CAD build for the part. Positions are in the model's coordinates, mm. A direction names the side the tool comes from. Coordinates: 2 decimals unless noted, no trailing zeros. Order: outer loops, then holes, each group sorted by start corner. A loop starts at its lowest first (then second) coordinate and runs counter-clockwise, first axis right, second up. Notation, with made-up numbers: (60.25, 24.5) - (95.25, 24.5) arc R9 cw to (95.25, 38.5) - close; hole circle Ø1 at (-37, 33.25). An arc over 180 degrees is marked (long way). Return JSON: item names as keys, results as strings.
from build123d import *

# Parameters (mm, degrees)
F1_R     = 1.5
F2_DEPTH = 3


with BuildPart() as f2:
    # F1 (on Top) → F2 (new body)
    with BuildSketch(Plane.XY):
        Polygon((19.1138070579, -24.5658658908), (30.8861929421, -3.8551877721), (24.5658658908, 19.1138070579), (3.8551877721, 30.8861929421), (-19.1138070579, 24.5658658908), (-30.8861929421, 3.8551877721), (-24.5658658908, -19.1138070579), (-3.8551877721, -30.8861929421), align=None)
        with BuildLine():
            add(Edge.make_bspline(
                [(-4.1445110049, -6.3067241031), (-5.9517399206, -7.2120212694), (-8.2435888807, -7.2120212694)],
                knots=[0, 0, 0, 1, 1, 1], degree=2))
            add(Edge.make_bspline(
                [(-8.2435888807, -7.2120212694), (-10.4546678333, -7.2120212694), (-11.6746314868, -6.0223463687)],
                knots=[0, 0, 0, 1, 1, 1], degree=2))
            add(Edge.make_bspline(
                [(-11.6746314868, -6.0223463687), (-12.8945951403, -4.832671468), (-12.8945951403, -2.665342936)],
                knots=[0, 0, 0, 1, 1, 1], degree=2))
            add(Edge.make_bspline(
                [(-12.8945951403, -2.665342936), (-12.8945951403, -0.49128357), (-12.0263175607, 1.3024836777)],
                knots=[0, 0, 0, 1, 1, 1], degree=2))
            add(Edge.make_bspline(
                [(-12.0263175607, 1.3024836777), (-11.1580399812, 3.0962509255), (-9.6755738036, 4.03688497)],
                knots=[0, 0, 0, 1, 1, 1], degree=2))
            add(Edge.make_bspline(
                [(-9.6755738036, 4.03688497), (-8.193107626, 4.9775190146), (-6.3219357878, 4.9775190146)],
                knots=[0, 0, 0, 1, 1, 1], degree=2))
            add(Edge.make_bspline(
                [(-6.3219357878, 4.9775190146), (-4.4574947836, 4.9775190146), (-3.4175809383, 4.1210203944)],
                knots=[0, 0, 0, 1, 1, 1], degree=2))
            add(Edge.make_bspline(
                [(-3.4175809383, 4.1210203944), (-2.377667093, 3.2645217742), (-2.377667093, 1.7702766373)],
                knots=[0, 0, 0, 1, 1, 1], degree=2))
            add(Edge.make_bspline(
                [(-2.377667093, 1.7702766373), (-2.377667093, -0.1951268762), (-4.1327320455, -1.2619640573)],
                knots=[0, 0, 0, 1, 1, 1], degree=2))
            add(Edge.make_bspline(
                [(-4.1327320455, -1.2619640573), (-5.887796998, -2.3288012385), (-9.148886047, -2.3288012385)],
                knots=[0, 0, 0, 1, 1, 1], degree=2))
            Line((-9.148886047, -2.3288012385), (-9.687352763, -2.3288012385))
            Line((-9.687352763, -2.3288012385), (-9.7075452649, -2.5509187588))
            Line((-9.7075452649, -2.5509187588), (-9.7075452649, -2.7629400283))
            add(Edge.make_bspline(
                [(-9.7075452649, -2.7629400283), (-9.7075452649, -3.7187184492), (-9.1657131319, -4.2706468331)],
                knots=[0, 0, 0, 1, 1, 1], degree=2))
            add(Edge.make_bspline(
                [(-9.1657131319, -4.2706468331), (-8.6238809989, -4.8225752171), (-7.6142559063, -4.8225752171)],
                knots=[0, 0, 0, 1, 1, 1], degree=2))
            add(Edge.make_bspline(
                [(-7.6142559063, -4.8225752171), (-6.6988624891, -4.8225752171), (-5.9517399206, -4.622332907)],
                knots=[0, 0, 0, 1, 1, 1], degree=2))
            add(Edge.make_bspline(
                [(-5.9517399206, -4.622332907), (-5.2046173521, -4.422090597), (-4.1445110049, -3.9172780508)],
                knots=[0, 0, 0, 1, 1, 1], degree=2))
            Line((-4.1445110049, -3.9172780508), (-4.1445110049, -6.3067241031))
        make_face(mode=Mode.SUBTRACT)
        with BuildLine():
            Line((9.8354311099, -0.2994548025), (8.4354176482, -7))
            Line((8.4354176482, -7), (5.2719256916, -7))
            Line((5.2719256916, -7), (6.712324157, -0.1311839537))
            add(Edge.make_bspline(
                [(6.712324157, -0.1311839537), (6.8805950057, 0.582284445), (6.8805950057, 1.1207511611)],
                knots=[0, 0, 0, 1, 1, 1], degree=2))
            add(Edge.make_bspline(
                [(6.8805950057, 1.1207511611), (6.8805950057, 2.4130712795), (5.7430840681, 2.4130712795)],
                knots=[0, 0, 0, 1, 1, 1], degree=2))
            add(Edge.make_bspline(
                [(5.7430840681, 2.4130712795), (4.7772093962, 2.4130712795), (3.9880191156, 1.2133001279)],
                knots=[0, 0, 0, 1, 1, 1], degree=2))
            add(Edge.make_bspline(
                [(3.9880191156, 1.2133001279), (3.1988288349, 0.0135289762), (2.7478629602, -2.1302416369)],
                knots=[0, 0, 0, 1, 1, 1], degree=2))
            Line((2.7478629602, -2.1302416369), (1.7146799488, -7))
            Line((1.7146799488, -7), (-1.4488120078, -7))
            Line((-1.4488120078, -7), (1.0415965538, 4.7587669112))
            Line((1.0415965538, 4.7587669112), (3.461331359, 4.7587669112))
            Line((3.461331359, 4.7587669112), (3.2392138386, 2.5813421283))
            Line((3.2392138386, 2.5813421283), (3.3031567611, 2.5813421283))
            add(Edge.make_bspline(
                [(3.3031567611, 2.5813421283), (4.8377869018, 4.9775190146), (7.0387696036, 4.9775190146)],
                knots=[0, 0, 0, 1, 1, 1], degree=2))
            add(Edge.make_bspline(
                [(7.0387696036, 4.9775190146), (8.4892643198, 4.9775190146), (9.283502726, 4.1008278926)],
                knots=[0, 0, 0, 1, 1, 1], degree=2))
            add(Edge.make_bspline(
                [(9.283502726, 4.1008278926), (10.0777411321, 3.2241367705), (10.0777411321, 1.5919095376)],
                knots=[0, 0, 0, 1, 1, 1], degree=2))
            add(Edge.make_bspline(
                [(10.0777411321, 1.5919095376), (10.0777411321, 0.8245944673), (9.8354311099, -0.2994548025)],
                knots=[0, 0, 0, 1, 1, 1], degree=2))
        make_face(mode=Mode.SUBTRACT)
        with BuildLine():
            add(Edge.make_bspline(
                [(18.7975365148, -5.4754661103), (17.3874268022, -7.2120212694), (15.4422157905, -7.2120212694)],
                knots=[0, 0, 0, 1, 1, 1], degree=2))
            add(Edge.make_bspline(
                [(15.4422157905, -7.2120212694), (13.894123982, -7.2120212694), (13.0056539005, -6.0913374167)],
                knots=[0, 0, 0, 1, 1, 1], degree=2))
            add(Edge.make_bspline(
                [(13.0056539005, -6.0913374167), (12.1171838191, -4.970653564), (12.1171838191, -2.9514033789)],
                knots=[0, 0, 0, 1, 1, 1], degree=2))
            add(Edge.make_bspline(
                [(12.1171838191, -2.9514033789), (12.1171838191, -0.8682102713), (12.8744026385, 1.0197886518)],
                knots=[0, 0, 0, 1, 1, 1], degree=2))
            add(Edge.make_bspline(
                [(12.8744026385, 1.0197886518), (13.6316214579, 2.9077875749), (14.8633640708, 3.9426532947)],
                knots=[0, 0, 0, 1, 1, 1], degree=2))
            add(Edge.make_bspline(
                [(14.8633640708, 3.9426532947), (16.0951066837, 4.9775190146), (17.5657939019, 4.9775190146)],
                knots=[0, 0, 0, 1, 1, 1], degree=2))
            add(Edge.make_bspline(
                [(17.5657939019, 4.9775190146), (18.5855152453, 4.9775190146), (19.3275896884, 4.5366493909)],
                knots=[0, 0, 0, 1, 1, 1], degree=2))
            add(Edge.make_bspline(
                [(19.3275896884, 4.5366493909), (20.0696641314, 4.0957797671), (20.4802450024, 3.2544255233)],
                knots=[0, 0, 0, 1, 1, 1], degree=2))
            Line((20.4802450024, 3.2544255233), (20.5643804267, 3.2544255233))
            Line((20.5643804267, 3.2544255233), (21.1634246483, 4.7587669112))
            Line((21.1634246483, 4.7587669112), (23.6033519553, 4.7587669112))
            Line((23.6033519553, 4.7587669112), (21.0994817258, -7))
            Line((21.0994817258, -7), (18.6898431716, -7))
            Line((18.6898431716, -7), (18.8379215185, -5.4754661103))
            Line((18.8379215185, -5.4754661103), (18.7975365148, -5.4754661103))
        make_face(mode=Mode.SUBTRACT)
        Polygon((-15.8494312445, -7), (-24.4413407821, -7), (-21.1937134011, 8.3765901595), (-17.9730093559, 8.3765901595), (-20.665342936, -4.3076664199), (-15.2806757757, -4.3076664199), align=None, mode=Mode.SUBTRACT)
        with Locations((0, 25)):
            Circle(F1_R, mode=Mode.SUBTRACT)
    extrude(amount=F2_DEPTH)


solid = f2.part
Item 1: Band-saw the part on C-C, the plane y = 14.5. List the corners of the cut face in (x, z), then the cut area to 3 significant figures.
Findings below:
{"outline": "(-24.84, 0) - (25.84, 0) - (25.84, 3) - (-24.84, 3) - close", "area": "152 mm²"}
Item 2: Drop flat-ended pins along their axis: P1, Ø1.2, axis at x = 19.5, z = 1.5, coming from the +Y side; P2, Ø1.5, axis at x = -0.5, z = 2, coming from the +Y side; P3, Ø0.7, axis at x = 22, z = 1, coming from the -Y side. Give the stop position or say it passes through.
Findings below:
{"P1": "stops at y = 22.33", "P2": "stops at y = 29.89", "P3": "stops at y = -20.1"}
Item 3: Band-saw the part on A-A, the plane x = 0. List the corners of the cut face in (y, z), then the cut area to 3 significant figures.
Findings below:
{"outline": "(-29.83, 0) - (-7, 0) - (-7, 3) - (-29.83, 3) - close; (-0.16, 0) - (23.5, 0) - (23.5, 3) - (-0.16, 3) - close; (26.5, 0) - (29.83, 0) - (29.83, 3) - (26.5, 3) - close", "area": "149 mm²"}
Item 4: Mould opens along X. For faces 1 (the flat face through (-24.918, 14.356, 1.479)), 2 (the flat face through (7, -7, 1)), 3 (the flat face through (7.47, -27.77, 1.48)) say: released by +X, released by -X, zero draft, split by the parting line, or undercut.
Findings below:
{"face 1": "released by -X", "face 2": "undercut", "face 3": "released by +X"}
Item 5: Which spindle directions (+Z, -Z, +X, -X, +Y, -Y) get a long thin tool onto all of the face, cutting with end or side? Do faces 4 (the flat face through (-0.4, 0.4, 3)), 5 (the flat face through (-18, -4.308, 1)). Say none if no direction does.
Findings below:
{"face 4": "+Z, +X, -X, +Y, -Y", "face 5": "+Z, -Z"}
Item 6: Band-saw the part on B-B, the plane z = 2.35. Count the separate pieces of the cut face and the enclosed holes in it, then the cut area to 3 significant figures.
Findings below:
{"separate pieces": "1", "enclosed holes": "5", "area": "2,400 mm²"}
Item 7: Wall check: L1, parallel to Y at x = -5.5, z = 0.55; L2, parallel to Y at x = -9, z = 2.4; L3, parallel to X at y = 0, z = 0.95. Give the ranges that are in metal, low to high. Write a range as [from, to].
Findings below:
{"L1": "y = [-29.95, -6.84], [-4.48, -1.86], [4.93, 28.31]", "L2": "y = [-27.96, -7.17], [-4.42, -2.33], [4.41, 27.35]", "L3": "x = [-29.83, -22.96], [-19.75, -12.53], [-2.83, 0.03], [3.37, 6.74], [9.9, 12.52], [22.59, 29.83]"}
